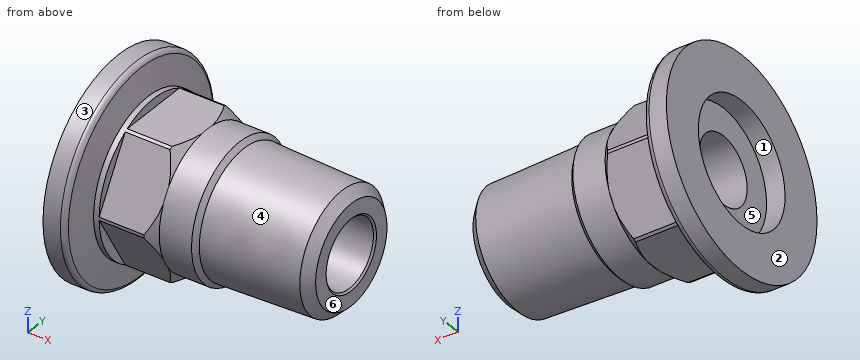
```python
from build123d import *

# Parameters (mm, degrees)
CHAMFER2_SIZE      = 1.27
CHAMFER2_SIZE2     = 1.311607448
SKETCH13_OUTSIDE_W = 42.75
SKETCH13_OUTSIDE_H = 42.75
CUT_EXTRUDE3_DEPTH = 7.62
CHAMFER3_SIZE      = 0.254


with BuildPart() as part:
    # Sketch1 → Revolve1 (revolve)
    with BuildSketch(Plane.XY, mode=Mode.PRIVATE) as revolve1_sk:
        with BuildLine():
            Line((2.463296835, 14.9987), (0, 14.9987))
            Line((0, 14.9987), (0, 8.636))
            Line((0, 8.636), (2.6162, 8.636))
            Line((2.6162, 8.636), (2.6162, 4.7625))
            Line((2.6162, 4.7625), (33.02, 4.7625))
            Line((33.02, 4.7625), (33.02, 8.382))
            Line((33.02, 8.382), (17.78, 8.858247176))
            Line((17.78, 8.858247176), (17.153656205, 9.525))
            Line((17.153656205, 9.525), (12.581656205, 9.525))
            Line((12.581656205, 9.525), (11.311656205, 10.795))
            Line((11.311656205, 10.795), (4.17437802, 10.795))
            Line((4.17437802, 10.795), (3.199332315, 14.433920112))
            ThreePointArc((3.199332315, 14.433920112), (2.927173044, 14.841235245), (2.463296835, 14.9987))
        make_face()
    revolve(revolve1_sk.sketch.rotate(Axis((0, 0, 0), (1, 0, 0)), 90), axis=Axis((0, 0, 0), (1, 0, 0)))

    # Chamfer2
    chamfer2_edges = [part.edges().sort_by_distance(p)[0] for p in [
        (33.02, 0, -8.382),
    ]]
    chamfer2_side = [part.faces().sort_by_distance(p)[0] for p in [
        (33.02, 0, -4.999578762),
    ]]
    chamfer(chamfer2_edges, length=CHAMFER2_SIZE, length2=CHAMFER2_SIZE2, reference=chamfer2_side[0])

    # Sketch13 outside → Cut-Extrude3 (cut)
    with BuildSketch(Plane(origin=(12.581656205, 0, 0), x_dir=(0, 0, -1), z_dir=(1, 0, 0))):
        Rectangle(SKETCH13_OUTSIDE_W, SKETCH13_OUTSIDE_H)
        Polygon((0, 10.925199144), (-9.4615, 5.462599572), (-9.4615, -5.462599572), (0, -10.925199144), (9.4615, -5.462599572), (9.4615, 5.462599572), align=None, mode=Mode.SUBTRACT)
    extrude(amount=-CUT_EXTRUDE3_DEPTH, mode=Mode.SUBTRACT)

    # Chamfer3
    chamfer3_edges = [part.edges().sort_by_distance(p)[0] for p in [
        (33.02, 0, -4.7625),
    ]]
    chamfer(chamfer3_edges, length=CHAMFER3_SIZE)


solid = part.part
```
Verification items for the finished model (mm, model axes). Face numbers are marked on the shaded views. A direction names the side the tool comes from. Coordinates: 2 decimals unless noted, no trailing zeros. Write each loop counter-clockwise with the first axis right and the second up, starting at its lowest first coordinate (ties: lowest second). Pieces come first, ordered by that corner, then holes. Notation, with made-up numbers: M -15,61.25 L 6,61.25 A35 ccw 6,95.25 Z; hole C 23.5,45.5 d1. An arc over 180 degrees is marked long. Answer as a JSON object with one key per item and string values. Group by question number.
(1) Gauge pin test, flat ends, axial feed: pin 1 (2 mm diameter, centred on x = 7.5, y = -1.5, fed in from -Z); pin 2 (5.5 mm diameter, centred on y = -7.5, z = 6.5, fed in from +X); pin 3 (3 mm diameter, centred on x = 15.5, z = 3, fed in from +Y); pin 4 (7.5 mm diameter, centred on y = 0, z = 0, fed in from -X). Record the tip position at first contact, or that the pin passes through.
(2) Cross-section at D-D, the plane x = 28.5. Record the cut outline in (y, z) (1 decimal).
(3) Cross-section at C-C, the plane x = 12. Record the cut outline in (y, z) (1 decimal), and give its area (3 significant figures).
(4) Cross-section at B-B, the plane x = 6. Record the cut outline in (y, z) (1 decimal), and give its area (3 significant figures).
(5) Material ranges on line 1 (Y direction, x = 2, z = 0); line 2 (Y direction, x = 22.5, z = 0); line 3 (Z direction, x = 25, y = -0.75), recorded low to high.
(6) Tool access check on the marked faces 4, 5 and 6. Record the directions out of +Z, -Z, +X, -X, +Y, -Y that give a thin tool (end or side, any length) a straight path to the whole face; none if there is none.
(7) Release check for a two-part mould opening along Z. For the marked faces 1, 2 and 3 record: +Z half, -Z half, draft (parallel to the pull), parting line (faces both ways), or undercut.
Reply:
{
 "1": {"pin 1": "z = -9.46", "pin 2": "x = 32.96", "pin 3": "y = 9.41", "pin 4": "through"},
 "2": {"outline": "C 0,0 d17; hole C 0,0 d9.5"},
 "3": {"outline": "M -10,-1.7 L -6.4,-7.8 A10.1 ccw -3.6,-9.5 L 3.6,-9.5 A10.1 ccw 6.4,-7.8 L 10,-1.7 A10.1 ccw 10,1.7 L 6.4,7.8 A10.1 ccw 3.6,9.5 L -3.6,9.5 A10.1 ccw -6.4,7.8 L -10,1.7 A10.1 ccw Z; hole C 0,0 d9.5", "area": "231 mm²"},
 "4": {"outline": "M -10.8,-0.2 L -5.6,-9.2 A10.8 ccw -5.2,-9.5 L 5.2,-9.5 A10.8 ccw 5.6,-9.2 L 10.8,-0.2 A10.8 ccw 10.8,0.2 L 5.6,9.2 A10.8 ccw 5.2,9.5 L -5.2,9.5 A10.8 ccw -5.6,9.2 L -10.8,0.2 A10.8 ccw Z; hole C 0,0 d9.5", "area": "239 mm²"},
 "5": {"line 1": "-15 to -8.64, 8.64 to 15", "line 2": "-8.71 to -4.76, 4.76 to 8.71", "line 3": "-8.6 to -4.7, 4.7 to 8.6"},
 "6": {"face 4": "+X", "face 5": "-X", "face 6": "+Z, -Z, +X, +Y, -Y"},
 "7": {"face 1": "undercut", "face 2": "draft", "face 3": "parting line"}
}
